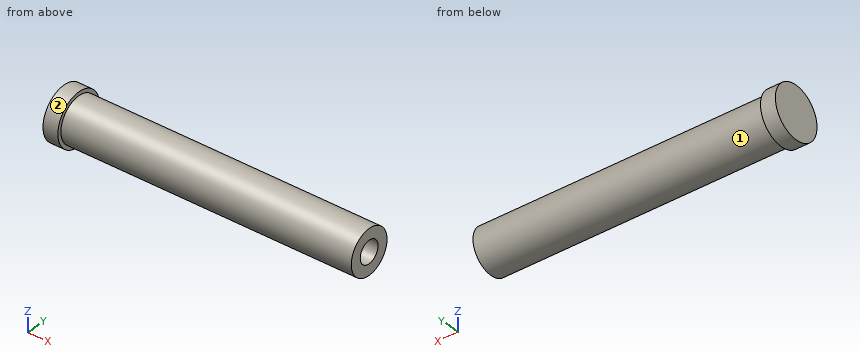
from build123d import *

# Parameters (mm, degrees)
SKETCH1_R           = 3.81
SKETCH1_R_2         = 1.905
BOSS_EXTRUDE1_DEPTH = 25.4
SKETCH2_R           = 4.445
BOSS_EXTRUDE2_DEPTH = 1.27


with BuildPart() as part:
    # Sketch1 → Boss-Extrude1 (new, symmetric)
    with BuildSketch(Plane(origin=(0, 0, 0), x_dir=(0, 0, -1), z_dir=(1, 0, 0))):
        Circle(SKETCH1_R)
        Circle(SKETCH1_R_2, mode=Mode.SUBTRACT)
    extrude(amount=BOSS_EXTRUDE1_DEPTH, both=True)

    # Sketch2 → Boss-Extrude2 (add, symmetric)
    with BuildSketch(Plane.ZY.offset(25.4)):
        Circle(SKETCH2_R)
    extrude(amount=BOSS_EXTRUDE2_DEPTH, both=True)


solid = part.part
Verification items for the finished model (mm, model axes). Face numbers are marked on the shaded views. A direction names the side the tool comes from. Coordinates: 2 decimals unless noted, no trailing zeros. Order: outer loops, then holes, each group sorted by start corner. A loop starts at its lowest first (then second) coordinate and runs counter-clockwise, first axis right, second up. Notation, with made-up numbers: M -9,-30 L 48,-30 A19 cw 48,-1 Z; hole C 83.5,-0.75 d11. An arc over 180 degrees is marked long. Return JSON: item names as keys, results as strings.
1) Access from +Z, -Z, +X, -X, +Y, -Y to the whole of each face (thin tool, end or side, straight path). Record for the marked faces 1 and 2.
Answer list:
{"face 1": "+X", "face 2": "+X, -X"}
2) Gauge pin test, flat ends, axial feed: pin 1 (1 mm diameter, centred on x = 12.5, z = -1, fed in from +Y); pin 2 (4 mm diameter, centred on x = -11, z = -3, fed in from +Y); pin 3 (2 mm diameter, centred on x = -11.5, y = 3, fed in from +Z). Record the tip position at first contact, or that the pin passes through.
Answer list:
{"pin 1": "y = 3.78", "pin 2": "y = 3.68", "pin 3": "z = 3.24"}
3) Cross-section at D-D, the plane z = 3. Record the boundary of the cut face in (x, y), and give its area (3 significant figures).
Answer list:
{"outline": "M -26.67,-3.28 L -24.13,-3.28 L -24.13,-2.35 L 25.4,-2.35 L 25.4,2.35 L -24.13,2.35 L -24.13,3.28 L -26.67,3.28 Z", "area": "249 mm2"}
4) Cross-section at C-C, the plane x = -5. Record the boundary of the cut face in (y, z) (3 decimals).
Answer list:
{"outline": "C 0,0 d7.62; hole C 0,0 d3.81"}
5) Thickness scan on L1, parallel to Y at x = -6.5, z = 0 (3 decimals); L2, parallel to X at y = 2, z = 3.5; L3, parallel to Z at x = 21, y = -0.5. Record the ranges inside material, lowest first. Write a range as [from, to].
Answer list:
{"L1": "[-3.81, -1.905], [1.905, 3.81]", "L2": "[-26.67, -24.13]", "L3": "[-3.78, -1.84], [1.84, 3.78]"}
6) Cross-section at A-A, the plane z = 0. Record the boundary of the cut face in (x, y) (3 decimals).
Answer list:
{"outline": "M -26.67,-4.445 L -24.13,-4.445 L -24.13,-3.81 L 25.4,-3.81 L 25.4,-1.905 L -24.13,-1.905 L -24.13,1.905 L 25.4,1.905 L 25.4,3.81 L -24.13,3.81 L -24.13,4.445 L -26.67,4.445 Z"}
